The drawing under review shows one solid part. Ordinate dimensions are in mm from its lowest x, y, z. Coordinates: 2 decimals unless noted, no trailing zeros. Write each loop counter-clockwise with the first axis right and the second up, starting at its lowest first coordinate (ties: lowest second). Pieces come first, ordered by that corner, then holes. Notation, with made-up numbers: (-12, -40) -> (37, -40) arc R5 ccw to (37, -31) -> close; hole circle Ø4 at (42.25, -28.5). An arc over 180 degrees is marked (long way). One line per item, written item: value. Start each with the question number.
1) Add section A-A (y = 23.5). State the section outline as (x, z) points.
2) For pin 1 Ø0.9 at (x, z) = (1, 25.5) entering from -Y; pin 2 Ø1.5 at (x, z) = (1.5, 1.5) entering from +Y; pin 3 Ø0.9 at (x, y) = (1.5, 2) entering from +Z, all flat-tipped, find the tip position at first contact; note any pin that passes through.
3) Add section D-D (z = 38.5). State the section outline as (x, y) points.
4) Add section B-B (x = 1.75). State the section outline as (y, z) points, and give its area (3 significant figures).
5) For probe 1 along Z at (x, y) = (2.6, 15.75); probe 2 along Z at (x, y) = (2.3, 23); probe 3 along Y at (x, z) = (2.55, 23.5), list the stretches that pass through material, from the lowest coordinate up. Write a range as from..to.
6) Add section C-C (y = 19.5). State the section outline as (x, z) points.
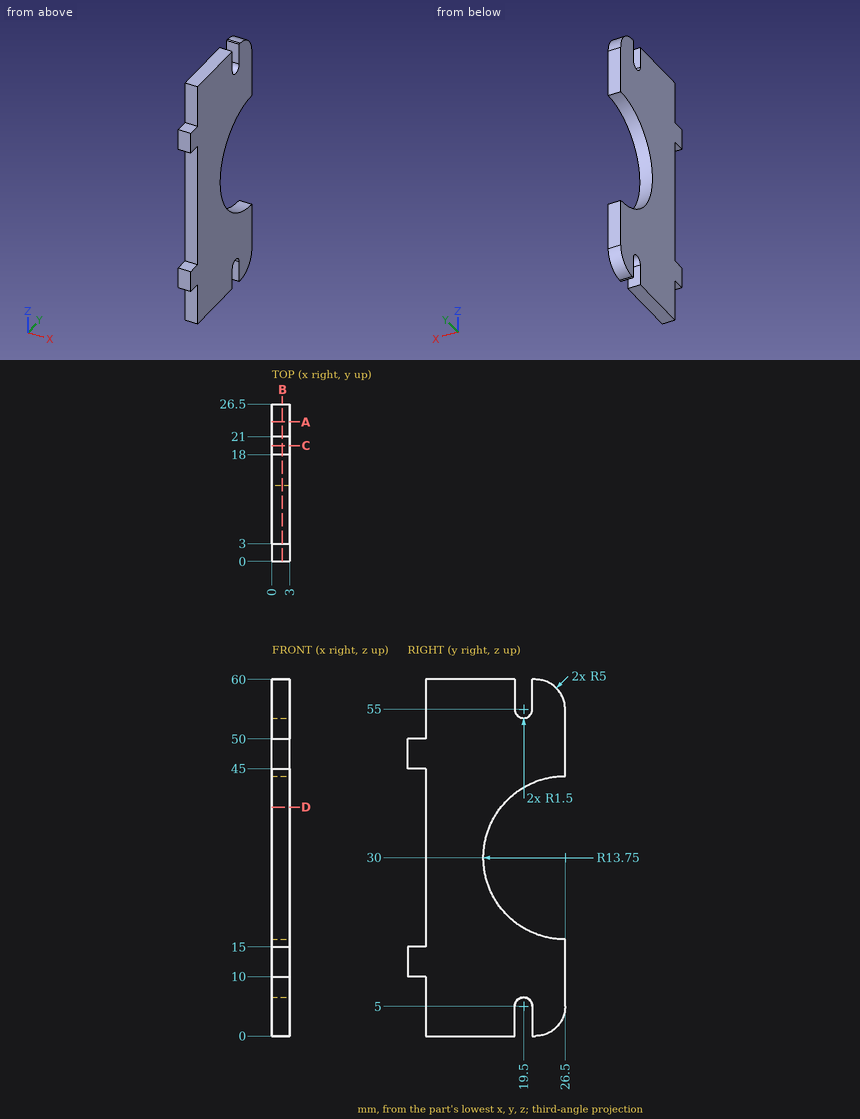
Numbers:
1. outline: (0, 0.42) -> (3, 0.42) -> (3, 16.58) -> (0, 16.58) -> close; (0, 43.42) -> (3, 43.42) -> (3, 59.58) -> (0, 59.58) -> close
2. pin 1: y = 3
2. pin 2: y = 25.68
2. pin 3: z = 50
3. outline: (0, 3) -> (3, 3) -> (3, 15.69) -> (0, 15.69) -> close
4. outline: (0, 10) -> (3, 10) -> (3, 0) -> (18, 0) -> (18, 5) arc R1.5 cw to (21, 5) -> (21, 0) -> (21.5, 0) arc R5 ccw to (26.5, 5) -> (26.5, 16.25) arc R13.75 cw to (26.5, 43.75) -> (26.5, 55) arc R5 ccw to (21.5, 60) -> (21, 60) -> (21, 55) arc R1.5 cw to (18, 55) -> (18, 60) -> (3, 60) -> (3, 50) -> (0, 50) -> (0, 45) -> (3, 45) -> (3, 15) -> (0, 15) -> close
4. area: 1,100 mm²
5. probe 1: 0..21.43, 38.57..60
5. probe 2: 0.23..16.7, 43.3..59.77
5. probe 3: 3..14.38
6. outline: (0, 6.5) -> (3, 6.5) -> (3, 18.17) -> (0, 18.17) -> close; (0, 41.83) -> (3, 41.83) -> (3, 53.5) -> (0, 53.5) -> close
